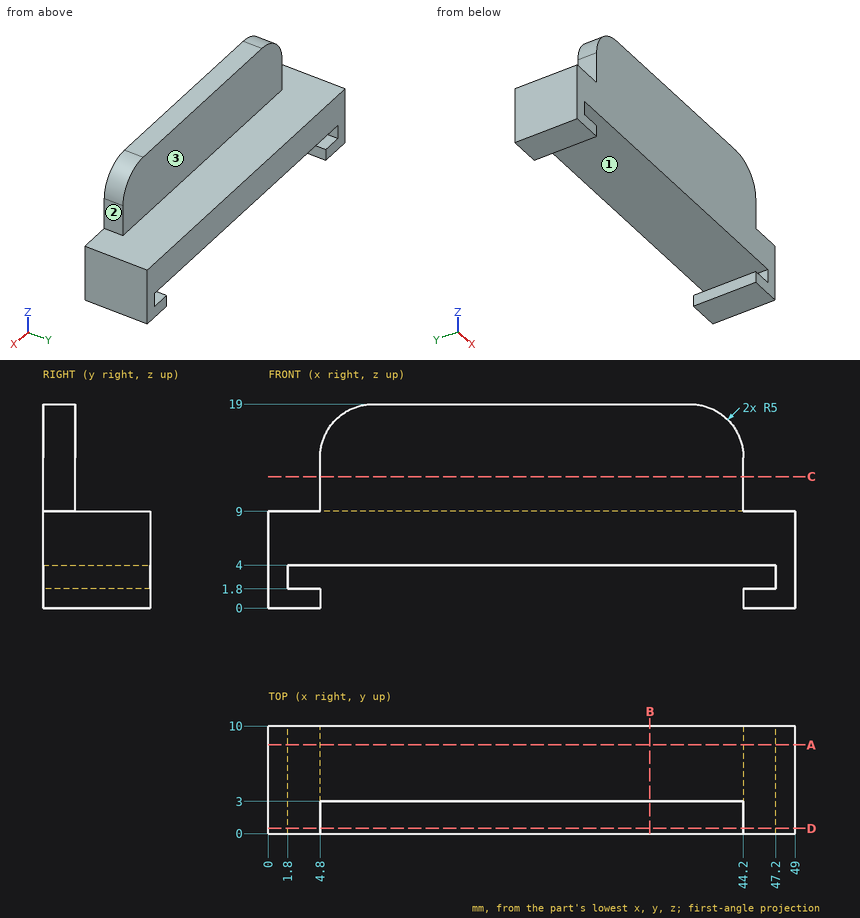
Answer from the drawing. Dimensions are ordinates in mm from the lowest x, y and z of the part. A direction names the side the tool comes from. Round coordinates to 2 decimals unless told otherwise and drop trailing zeros. Loops run counter-clockwise (first coordinate to the right, second up) from the corner with the lowest first, then second, coordinate; pieces in that order, holes last.
1) Given P1, Ø2.5, axis at y = 1.5, z = 12.5, coming from the -X side; P2, Ø2, axis at x = 15, y = 8, coming from the +Z side; P3, Ø2, axis at x = 32.5, z = 8, coming from the -Y side; P4, Ø3, axis at y = 3.5, z = 13.5, coming from the +X side, each flat-ended and moving along its own axis, determine where each tip first touches the part or whether it passes through.
Outcome:
P1: stops at x = 4.8
P2: stops at z = 9
P3: stops at y = 0
P4: stops at x = 44.2
2) A cutting plane is placed at D-D on y = 0.5. Determine the outline of the cut face in (x, z).
Outcome:
outline: (0, 0) - (4.8, 0) - (4.8, 1.8) - (1.8, 1.8) - (1.8, 4) - (47.2, 4) - (47.2, 1.8) - (44.2, 1.8) - (44.2, 0) - (49, 0) - (49, 9) - (44.2, 9) - (44.2, 14) arc R5 ccw to (39.2, 19) - (9.8, 19) arc R5 ccw to (4.8, 14) - (4.8, 9) - (0, 9) - close
3) A cutting plane is placed at B-B on x = 35.5. Determine the outline of the cut face in (y, z), plus the area to 3 significant figures.
Outcome:
outline: (0, 4) - (10, 4) - (10, 9) - (3, 9) - (3, 19) - (0, 19) - close
area: 80.0 mm2
4) Consider line 1 (Z direction, x = 44.5, y = 7.5); line 2 (Z direction, x = 5, y = 4.75); line 3 (Y direction, x = 39, z = 14.75). Determine where each line is inside the solid, lowest interval first.
Outcome:
line 1: z = 0 to 1.8, 4 to 9
line 2: z = 4 to 9
line 3: y = 0 to 3
5) A cutting plane is placed at A-A on y = 8.25. Determine the outline of the cut face in (x, z), plus the area to 3 significant figures.
Outcome:
outline: (0, 0) - (4.8, 0) - (4.8, 1.8) - (1.8, 1.8) - (1.8, 4) - (47.2, 4) - (47.2, 1.8) - (44.2, 1.8) - (44.2, 0) - (49, 0) - (49, 9) - (0, 9) - close
area: 270 mm2
6) A cutting plane is placed at C-C on z = 12.25. Determine the outline of the cut face in (x, y), plus the area to 3 significant figures.
Outcome:
outline: (4.8, 0) - (44.2, 0) - (44.2, 3) - (4.8, 3) - close
area: 118 mm2
7) For the marked faces 1, 2 and 3, determine the directions among +Z, -Z, +X, -X, +Y, -Y from which every point of the face is accessible in a straight line to the end or side of a thin tool.
Outcome:
face 1: +Y, -Y
face 2: +Z, +X, +Y, -Y
face 3: +Z, +X, -X, +Y
